Could you check a few things on this model? Use its own coordinates, in mm. A direction names the side the tool comes from. Give positions to 0.01 mm unless a question says otherwise; leave off trailing zeros. Order: outer loops, then holes, each group sorted by start corner. A loop starts at its lowest first (then second) coordinate and runs counter-clockwise, first axis right, second up. Notation, with made-up numbers: M 68,53 L 78,53 A24 ccw 78,83 Z; hole C -2,-28 d5. An arc over 180 degrees is marked long. Use a Markdown table: item, result. Add a question column.
Item 1: I'm going to push flat-ended pins straight in: pin 1 Ø4 at (x, y) = (3, -7.5) entering from +Z; pin 2 Ø18 at (x, y) = (8, 4) entering from -Z; pin 3 Ø5.5 at (x, y) = (44, 0.5) entering from +Z. Where does each tip first touch, or does it pass through?
Item 2: If we mould it in two halves opening along X, with no side actions, what happens to faces 1 (the face through (15.376, 2.009, 11.479)), 2 (the face through (2, 0, 0)), 3 (the face through (15.65, 12.91, 11.48)), 4 (the face through (17.402, 19.639, 5.07))? For each: released by +X, released by -X, zero draft, split by the parting line, or undercut.
Item 3: Suppose I cut it at D-D on z = -10.5. Write out the boundary of the cut face in (x, y), plus the area to 3 significant figures.
Item 4: For faces 5 (the face through (2.404, 14.806, 11.479)), 6 (the face through (-4.49, 25.68, 11.48)), 7 (the face through (-10.864, 17.246, 11.479)), which set-ups out of +Z, -Z, +X, -X, +Y, -Y let a thin tool reach every point of the face, with its end or its side?
Item 5: Suppose I cut it at B-B on z = 2.5. Write out the boundary of the cut face in (x, y).
Item 6: If I drill on L1, parallel to X at y = 1, z = 7; L2, parallel to Z at x = 20, y = -0.5; L3, parallel to Y at x = -15, z = 11.25, over which ranges is the centre line in solid material (lowest first)? Write a range as from..to.
Item 7: Suppose I cut it at C-C on x = 35. Write out the boundary of the cut face in (y, z).
Item 8: Suppose I cut it at A-A on z = 7.5. Write out the boundary of the cut face in (x, y), plus the area to 3 significant figures.
from build123d import *

# Parameters (mm, degrees)
EXTRUDE_1_DEPTH     = 10
EXTRUDE_2_DEPTH     = 3
CUT_EXTRUDE_1_DEPTH = 60.160797831
CUT_EXTRUDE_START   = -5
CUT_EXTRUDE_2_DEPTH = 5
SKETCH_6_R          = 4.2
EXTRUDE_3_DEPTH     = 15
SKETCH_7_R          = 8
EXTRUDE_4_DEPTH     = 5
EXTRUDE_6_DEPTH     = 7


with BuildPart() as part:
    # 草图1 → 凸台-拉伸1 (new body)
    with BuildSketch(Plane.XY):
        with BuildLine():
            Line((12.857142857, 27.105237087), (41.428571429, 13.552618544))
            ThreePointArc((41.428571429, 13.552618544), (50, 0), (41.428571429, -13.552618544))
            Line((41.428571429, -13.552618544), (12.857142857, -27.105237087))
            ThreePointArc((12.857142857, -27.105237087), (-30, 0), (12.857142857, 27.105237087))
        make_face()
    extrude(amount=EXTRUDE_1_DEPTH)

    # 草图2 → 凸台-拉伸2 (add)
    with BuildSketch(Plane.XY.offset(10)):
        with BuildLine():
            Line((23.957377721, 0.209887463), (16.67642367, 1.377277592))
            ThreePointArc((16.67642367, 1.377277592), (15.360611936, 2.023540765), (14.633319135, 3.296357245))
            ThreePointArc((14.633319135, 3.296357245), (14.013905466, 5.34887405), (13.10820337, 7.292119336))
            ThreePointArc((13.10820337, 7.292119336), (12.830802367, 8.073818452), (12.824431404, 8.903254546))
            ThreePointArc((12.824431404, 8.903254546), (13.010978482, 9.528656304), (13.353035008, 10.084466078))
            Line((13.353035008, 10.084466078), (18.004501541, 15.806262185))
            ThreePointArc((18.004501541, 15.806262185), (20.022964964, 16.728032941), (21.979510308, 15.681234856))
            ThreePointArc((21.979510308, 15.681234856), (25.225029838, 9.62797329), (26.838176005, 2.95166203))
            ThreePointArc((26.838176005, 2.95166203), (26.85239584, 2.616563886), (26.821632235, 2.282578003))
            ThreePointArc((26.821632235, 2.282578003), (25.818773244, 0.6530262), (23.957377721, 0.209887463))
        make_face()
        with BuildLine():
            Line((15.409921311, -6.521834496), (22.690875361, -7.689224625))
            ThreePointArc((22.690875361, -7.689224625), (24.498383964, -8.976379847), (24.570102902, -11.194196862))
            ThreePointArc((24.570102902, -11.194196862), (20.950584375, -17.031530006), (15.975302304, -21.766711196))
            ThreePointArc((15.975302304, -21.766711196), (15.692208716, -21.946575006), (15.387586654, -22.086925885))
            ThreePointArc((15.387586654, -22.086925885), (13.4749239, -22.033200424), (12.160456735, -20.642753983))
            Line((12.160456735, -20.642753983), (9.530969218, -13.753567747))
            ThreePointArc((9.530969218, -13.753567747), (9.432743676, -12.290909771), (10.171388682, -11.02464749))
            ThreePointArc((10.171388682, -11.02464749), (11.639213542, -9.461961114), (12.869262278, -7.705977448))
            ThreePointArc((12.869262278, -7.705977448), (13.407533068, -7.074891575), (14.122660315, -6.654656112))
            ThreePointArc((14.122660315, -6.654656112), (14.757547664, -6.503509741), (15.409921311, -6.521834496))
        make_face()
        with BuildLine():
            Line((2.056886303, -16.606300573), (4.68637382, -23.49548681))
            ThreePointArc((4.68637382, -23.49548681), (4.475419, -25.704412788), (2.590592594, -26.875431718))
            ThreePointArc((2.590592594, -26.875431718), (-4.274445463, -26.659503296), (-10.862873701, -24.718373226))
            ThreePointArc((-10.862873701, -24.718373226), (-11.160187124, -24.563138893), (-11.434045581, -24.369503888))
            ThreePointArc((-11.434045581, -24.369503888), (-12.343849344, -22.686226624), (-11.796920986, -20.852641446))
            Line((-11.796920986, -20.852641446), (-7.145454452, -15.130845339))
            ThreePointArc((-7.145454452, -15.130845339), (-5.92786826, -14.314450537), (-4.461930453, -14.321004735))
            ThreePointArc((-4.461930453, -14.321004735), (-2.374691924, -14.810835164), (-0.238941092, -14.998096784))
            ThreePointArc((-0.238941092, -14.998096784), (0.576730701, -15.148710026), (1.298228911, -15.557910658))
            ThreePointArc((1.298228911, -15.557910658), (1.746569183, -16.032166046), (2.056886303, -16.606300573))
        make_face()
        with BuildLine():
            Line((-13.353035008, -10.084466078), (-18.004501541, -15.806262185))
            ThreePointArc((-18.004501541, -15.806262185), (-20.022964964, -16.728032941), (-21.979510308, -15.681234856))
            ThreePointArc((-21.979510308, -15.681234856), (-25.225029838, -9.62797329), (-26.838176005, -2.95166203))
            ThreePointArc((-26.838176005, -2.95166203), (-26.85239584, -2.616563886), (-26.821632235, -2.282578003))
            ThreePointArc((-26.821632235, -2.282578003), (-25.818773244, -0.6530262), (-23.957377721, -0.209887463))
            Line((-23.957377721, -0.209887463), (-16.67642367, -1.377277592))
            ThreePointArc((-16.67642367, -1.377277592), (-15.360611936, -2.023540765), (-14.633319135, -3.296357245))
            ThreePointArc((-14.633319135, -3.296357245), (-14.013905466, -5.34887405), (-13.10820337, -7.292119336))
            ThreePointArc((-13.10820337, -7.292119336), (-12.830802367, -8.073818452), (-12.824431404, -8.903254546))
            ThreePointArc((-12.824431404, -8.903254546), (-13.010978482, -9.528656304), (-13.353035008, -10.084466078))
        make_face()
        with BuildLine():
            Line((-15.409921311, 6.521834496), (-22.690875361, 7.689224625))
            ThreePointArc((-22.690875361, 7.689224625), (-24.498383964, 8.976379847), (-24.570102902, 11.194196862))
            ThreePointArc((-24.570102902, 11.194196862), (-20.950584375, 17.031530006), (-15.975302304, 21.766711196))
            ThreePointArc((-15.975302304, 21.766711196), (-15.692208716, 21.946575006), (-15.387586654, 22.086925885))
            ThreePointArc((-15.387586654, 22.086925885), (-13.4749239, 22.033200424), (-12.160456735, 20.642753983))
            Line((-12.160456735, 20.642753983), (-9.530969218, 13.753567747))
            ThreePointArc((-9.530969218, 13.753567747), (-9.432743676, 12.290909771), (-10.171388682, 11.02464749))
            ThreePointArc((-10.171388682, 11.02464749), (-11.639213542, 9.461961114), (-12.869262278, 7.705977448))
            ThreePointArc((-12.869262278, 7.705977448), (-13.407533068, 7.074891575), (-14.122660315, 6.654656112))
            ThreePointArc((-14.122660315, 6.654656112), (-14.757547664, 6.503509741), (-15.409921311, 6.521834496))
        make_face()
        with BuildLine():
            Line((-2.056886303, 16.606300573), (-4.68637382, 23.49548681))
            ThreePointArc((-4.68637382, 23.49548681), (-4.475419, 25.704412788), (-2.590592594, 26.875431718))
            ThreePointArc((-2.590592594, 26.875431718), (4.274445463, 26.659503296), (10.862873701, 24.718373226))
            ThreePointArc((10.862873701, 24.718373226), (11.160187124, 24.563138893), (11.434045581, 24.369503888))
            ThreePointArc((11.434045581, 24.369503888), (12.343849344, 22.686226624), (11.796920986, 20.852641446))
            Line((11.796920986, 20.852641446), (7.145454452, 15.130845339))
            ThreePointArc((7.145454452, 15.130845339), (5.92786826, 14.314450537), (4.461930453, 14.321004735))
            ThreePointArc((4.461930453, 14.321004735), (2.374691924, 14.810835164), (0.238941092, 14.998096784))
            ThreePointArc((0.238941092, 14.998096784), (-0.576730701, 15.148710026), (-1.298228911, 15.557910658))
            ThreePointArc((-1.298228911, 15.557910658), (-1.746569183, 16.032166046), (-2.056886303, 16.606300573))
        make_face()
    extrude(amount=EXTRUDE_2_DEPTH)

    # 草图4 → 切除-拉伸1 (cut, through all)
    with BuildSketch(Plane.XY.offset(10)):
        with BuildLine():
            ThreePointArc((26.313917142, -4.219035984), (24.945941386, -2.328628005), (23.055533406, -3.696603761))
            ThreePointArc((23.055533406, -3.696603761), (24.423509162, -5.587011741), (26.313917142, -4.219035984))
        make_face()
        with BuildLine():
            ThreePointArc((9.503166229, -24.89803871), (10.456319685, -22.768132964), (8.326413938, -21.814979508))
            ThreePointArc((8.326413938, -21.814979508), (7.373260482, -23.944885255), (9.503166229, -24.89803871))
        make_face()
        with BuildLine():
            ThreePointArc((-16.810750913, -20.679002726), (-14.489621701, -20.439504959), (-14.729119468, -18.118375747))
            ThreePointArc((-14.729119468, -18.118375747), (-17.05024868, -18.357873514), (-16.810750913, -20.679002726))
        make_face()
        with BuildLine():
            ThreePointArc((-26.313917142, 4.219035984), (-24.945941386, 2.328628005), (-23.055533406, 3.696603761))
            ThreePointArc((-23.055533406, 3.696603761), (-24.423509162, 5.587011741), (-26.313917142, 4.219035984))
        make_face()
        with BuildLine():
            ThreePointArc((-9.503166229, 24.89803871), (-10.456319685, 22.768132964), (-8.326413938, 21.814979508))
            ThreePointArc((-8.326413938, 21.814979508), (-7.373260482, 23.944885255), (-9.503166229, 24.89803871))
        make_face()
        with BuildLine():
            ThreePointArc((16.810750913, 20.679002726), (14.489621701, 20.439504959), (14.729119468, 18.118375747))
            ThreePointArc((14.729119468, 18.118375747), (17.05024868, 18.357873514), (16.810750913, 20.679002726))
        make_face()
    extrude(amount=-CUT_EXTRUDE_1_DEPTH, mode=Mode.SUBTRACT)

    # 草图5 → 切除-拉伸2 (cut)
    with BuildSketch(Plane.XY.offset(10).offset(CUT_EXTRUDE_START)):
        with BuildLine():
            Line((41.428571429, 13.552618544), (12.857142857, 27.105237087))
            ThreePointArc((12.857142857, 27.105237087), (30, 0), (12.857142857, -27.105237087))
            Line((12.857142857, -27.105237087), (41.428571429, -13.552618544))
            ThreePointArc((41.428571429, -13.552618544), (50, 0), (41.428571429, 13.552618544))
        make_face()
    extrude(amount=CUT_EXTRUDE_2_DEPTH, mode=Mode.SUBTRACT)

    # 草图6 → 凸台-拉伸3 (add)
    with BuildSketch(Plane(origin=(0, 0, 0), x_dir=(-1, 0, 0), z_dir=(0, 0, -1))):
        with Locations(Location((-35, 0, 0), (0, 0, 180))):
            Circle(SKETCH_6_R)
    extrude(amount=EXTRUDE_3_DEPTH)

    # 草图7 → 凸台-拉伸4 (add)
    with BuildSketch(Plane(origin=(0, 0, 0), x_dir=(-1, 0, 0), z_dir=(0, 0, -1))):
        with Locations(Location((-35, 0, 0), (0, 0, 180))):
            Circle(SKETCH_7_R)
    extrude(amount=EXTRUDE_4_DEPTH)

    # 草图8 → 凸台-拉伸6 (add)
    with BuildSketch(Plane.XY.offset(5)):
        with BuildLine():
            ThreePointArc((42.632129039, 5.612626265), (42.907933699, 2.812334557), (43, 0))
            Line((43, 0), (47.5, 0))
            ThreePointArc((47.5, 0), (47.398298854, 3.106648638), (47.093630915, 6.19999413))
            Line((47.093630915, 6.19999413), (42.632129039, 5.612626265))
        make_face()
        with BuildLine():
            Line((47.5, 0), (43, 0))
            ThreePointArc((43, 0), (42.907933699, -2.812334557), (42.632129039, -5.612626265))
            Line((42.632129039, -5.612626265), (47.093630915, -6.19999413))
            ThreePointArc((47.093630915, -6.19999413), (47.398298854, -3.106648638), (47.5, 0))
        make_face()
    extrude(amount=EXTRUDE_6_DEPTH)


solid = part.part
Findings below:
| question | item | result |
|---|---|---|
| 1 | pin 1 | stops at z = 10 |
| 1 | pin 2 | stops at z = 0 |
| 1 | pin 3 | stops at z = 12 |
| 2 | face 1 | released by -X |
| 2 | face 2 | zero draft |
| 2 | face 3 | undercut |
| 2 | face 4 | undercut |
| 3 | outline | C 35,0 d8.4 |
| 3 | area | 55.4 mm^2 |
| 4 | face 5 | +Z |
| 4 | face 6 | +Z, -X |
| 4 | face 7 | +Z, +Y |
| 5 | outline | M 12.86,-27.11 L 41.43,-13.55 A15 ccw 41.43,13.55 L 12.86,27.11 A30 ccw long Z; hole C -24.68,3.96 d3.3; hole C -15.77,-19.4 d3.3; hole C -8.91,23.36 d3.3; hole C 8.91,-23.36 d3.3; hole C 15.77,19.4 d3.3; hole C 24.68,-3.96 d3.3 |
| 6 | L1 | x = -29.98..29.98, 42.99..47.49 |
| 6 | L2 | z = 0..10 |
| 6 | L3 | y = -12.11..-2.45, 6.49..22.2 |
| 7 | outline | M -16.6,0 L -8,0 L -8,-5 L -4.2,-5 L -4.2,-15 L 4.2,-15 L 4.2,-5 L 8,-5 L 8,0 L 16.6,0 L 16.6,5 L -16.6,5 Z |
| 8 | outline | C 0,0 d60; M 42.63,-5.61 L 47.09,-6.2 A47.5 ccw 47.09,6.2 L 42.63,5.61 A43 cw Z; hole C -24.68,3.96 d3.3; hole C -15.77,-19.4 d3.3; hole C -8.91,23.36 d3.3; hole C 8.91,-23.36 d3.3; hole C 15.77,19.4 d3.3; hole C 24.68,-3.96 d3.3 |
| 8 | area | 2,830 mm^2 |
